The model under review builds one solid part; all positions refer to its coordinate system, in mm. A direction names the side the tool comes from. Give positions to 0.01 mm unless a question says otherwise; leave off trailing zeros. Loops run counter-clockwise (first coordinate to the right, second up) from the corner with the lowest first, then second, coordinate; pieces in that order, holes last. Notation, with made-up numbers: (-11.5, -17) - (22.5, -17) arc R23 cw to (22.5, 15) - close; hole circle Ø9 at (31.5, 37.25). An arc over 180 degrees is marked (long way). Return JSON: item names as keys, results as strings. Group by question number.
```python
from build123d import *

# Parameters (mm, degrees)
BOSS_EXTRUDE1_DEPTH = 25.4
CUT_EXTRUDE1_REACH  = 78.2
SKETCH2_R           = 3.175
CUT_EXTRUDE2_REACH  = 74.122
SKETCH3_R           = 3.175
FILLET1_R           = 3.175
FILLET2_R           = 3.175


with BuildPart() as part:
    # Sketch1 → Boss-Extrude1 (new body)
    with BuildSketch(Plane(origin=(0, 0, 0), x_dir=(0, 0, -1), z_dir=(1, 0, 0))):
        Polygon((0, 0), (50.8, 0), (50.8, 6.35), (6.35, 6.35), (6.35, 50.8), (0, 50.8), align=None)
    extrude(amount=BOSS_EXTRUDE1_DEPTH)

    # Sketch2 → Cut-Extrude1 (cut, up to next)
    with BuildSketch(Plane.XY, mode=Mode.PRIVATE) as cut_extrude1_sk1:
        with Locations((12.7, 29.21)):
            Circle(SKETCH2_R)
    cut_extrude1_tool1 = extrude(cut_extrude1_sk1.sketch, amount=-CUT_EXTRUDE1_REACH, mode=Mode.PRIVATE) & part.part
    add(cut_extrude1_tool1.solids().sort_by_distance((12.7, 29.21, 0))[0], mode=Mode.SUBTRACT)

    # Sketch3 → Cut-Extrude2 (cut, up to next)
    with BuildSketch(Plane(origin=(0, 6.35, 0), x_dir=(1, 0, 0), z_dir=(0, 1, 0)), mode=Mode.PRIVATE) as cut_extrude2_sk1:
        with Locations(Location((12.7, 29.21, 0), (0, 0, 270))):
            Circle(SKETCH3_R)
    cut_extrude2_tool1 = extrude(cut_extrude2_sk1.sketch, amount=-CUT_EXTRUDE2_REACH, mode=Mode.PRIVATE) & part.part
    add(cut_extrude2_tool1.solids().sort_by_distance((12.7, 6.35, -29.21))[0], mode=Mode.SUBTRACT)

    # Fillet1
    fillet1_edges = [part.edges().sort_by_distance(p)[0] for p in [
        (12.7, 6.35, -6.35),
    ]]
    fillet(fillet1_edges, radius=FILLET1_R)

    # Fillet2
    fillet2_edges = [part.edges().sort_by_distance(p)[0] for p in [
        (12.7, 50.8, -6.35),
        (12.7, 6.35, -50.8),
    ]]
    fillet(fillet2_edges, radius=FILLET2_R)


solid = part.part
```
1) We need section A-A, the plane z = -29.21. Write out the cut boundary in (x, y) (3 decimals), plus the area to 3 significant figures.
2) To check wall thickness, follow line 1 (X direction, y = 4, z = -29); line 2 (Y direction, x = 4.5, z = -9.5); line 3 (Z direction, x = 1.5, y = 11). State the ranges of each line that lie inside material, in increasing order.
3) Tool access review of faces 4 (the face through (12.5, 25.8, 0)), 5 (the face through (13, 24, -6.35)): name each direction out of +Z, -Z, +X, -X, +Y, -Y from which nothing blocks a thin tool from reaching the whole face with its end or side.
4) We need section D-D, the plane x = 21.5. Write out the cut boundary in (y, z) (3 decimals), plus the area to 3 significant figures.
5) We need section B-B, the plane y = 29.21. Write out the cut boundary in (x, z) (3 decimals), plus the area to 3 significant figures.
6) Draft analysis for pull direction X (two halves, no side actions). For faces 1 (the face through (0, 5, -16)), 2 (the face through (13, 6.35, -25)), 3 (the face through (10.18, 27.28, -3.13)), state which applies: +X half, -X half, draft (parallel to the pull), parting line (faces both ways), or undercut.
7) For pin 1 Ø8 at (x, y) = (4, 22) entering from +Z; pin 2 Ø2 at (x, z) = (17, -35.5) entering from +Y; pin 3 Ø4 at (x, y) = (10, 27.5) entering from -Z, all flat-tipped, find the tip position at first contact; note any pin that passes through.
8) We need section C-C, the plane x = 12.7. Write out the cut boundary in (y, z) (3 decimals).
Findings:
{
 "1": {"outline": "(0, 0) - (9.525, 0) - (9.525, 6.35) - (0, 6.35) - close; (15.875, 0) - (25.4, 0) - (25.4, 6.35) - (15.875, 6.35) - close", "area": "121 mm^2"},
 "2": {"line 1": "x = 0 to 9.53, 15.87 to 25.4", "line 2": "y = 0 to 6.35", "line 3": "z = -6.35 to 0"},
 "3": {"face 4": "+Z, +X, -X, +Y, -Y", "face 5": "-Z, +X, -X, +Y"},
 "4": {"outline": "(0, -50.8) - (3.175, -50.8) arc R3.175 ccw to (6.35, -47.625) - (6.35, -9.525) arc R3.175 cw to (9.525, -6.35) - (47.625, -6.35) arc R3.175 ccw to (50.8, -3.175) - (50.8, 0) - (0, 0) - close", "area": "603 mm^2"},
 "5": {"outline": "(0, -6.35) - (9.525, -6.35) - (9.525, 0) - (0, 0) - close; (15.875, -6.35) - (25.4, -6.35) - (25.4, 0) - (15.875, 0) - close", "area": "121 mm^2"},
 "6": {"face 1": "-X half", "face 2": "draft", "face 3": "undercut"},
 "7": {"pin 1": "stops at z = 0", "pin 2": "stops at y = 6.35", "pin 3": "stops at z = -6.35"},
 "8": {"outline": "(0, -50.8) - (3.175, -50.8) arc R3.175 ccw to (6.35, -47.625) - (6.35, -32.385) - (0, -32.385) - close; (0, -26.035) - (6.35, -26.035) - (6.35, -9.525) arc R3.175 cw to (9.525, -6.35) - (26.035, -6.35) - (26.035, 0) - (0, 0) - close; (32.385, -6.35) - (47.625, -6.35) arc R3.175 ccw to (50.8, -3.175) - (50.8, 0) - (32.385, 0) - close"}
}
